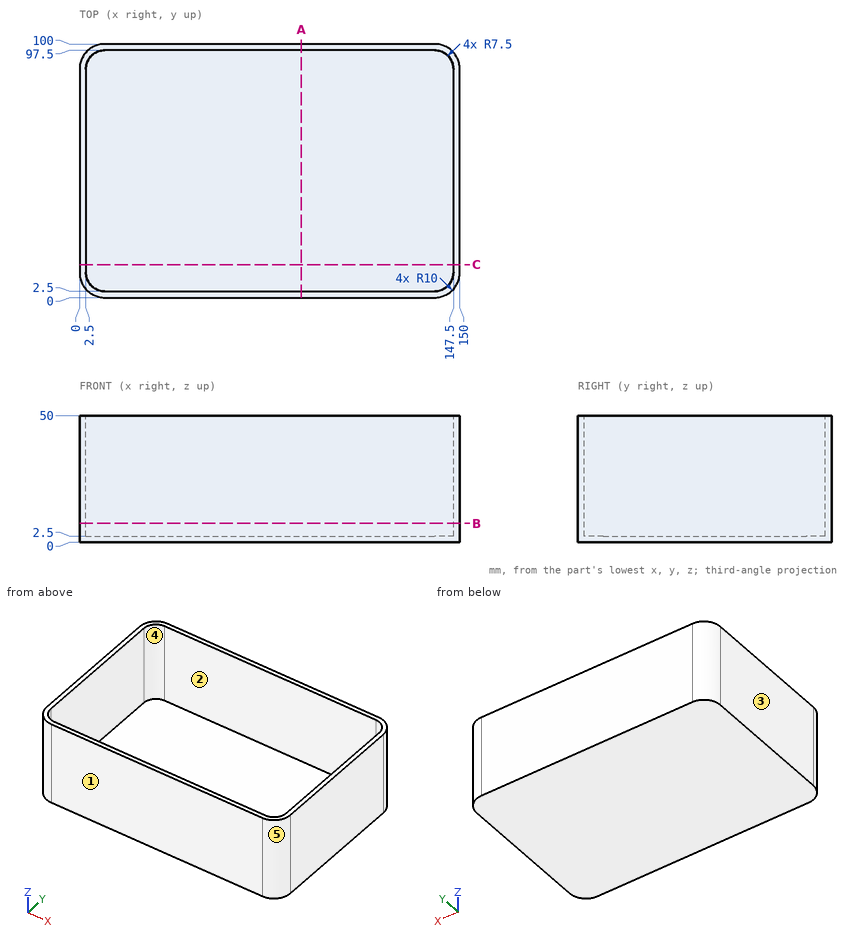
Here's the drawing with two shaded views (mm, measured from the low corner). I have some questions. A direction names the side the tool comes from. Round coordinates to 2 decimals unless told otherwise and drop trailing zeros. Order: outer loops, then holes, each group sorted by start corner. A loop starts at its lowest first (then second) coordinate and runs counter-clockwise, first axis right, second up. Notation, with made-up numbers: M 70,65 L 107,65 A18 cw 107,82 Z; hole C 23,67 d6. An arc over 180 degrees is marked long. Answer in a Markdown table with one row per item.
Item 1: For the marked faces 4 and 5, which set-ups out of +Z, -Z, +X, -X, +Y, -Y let a thin tool reach every point of the face, with its end or its side?
A:
| item | result |
|---|---|
| face 4 | +Z |
| face 5 | +Z, -Z, +X, -Y |
Item 2: Imagine slicing it at B-B, the plane z = 7.5. Write out the boundary of the cut face in (x, y), and give its area (3 significant figures).
A:
| item | result |
|---|---|
| outline | M 0,10 A10 ccw 10,0 L 140,0 A10 ccw 150,10 L 150,90 A10 ccw 140,100 L 10,100 A10 ccw 0,90 Z; hole M 2.5,10 A7.5 ccw 10,2.5 L 140,2.5 A7.5 ccw 147.5,10 L 147.5,90 A7.5 ccw 140,97.5 L 10,97.5 A7.5 ccw 2.5,90 Z |
| area | 1,190 mm2 |
Item 3: If I drill on L1, parallel to Y at x = 39, z = 26; L2, parallel to X at y = 79.5, z = 30; L3, parallel to Z at x = 118, y = 58, over which ranges is the centre line in solid material (lowest first)? Write a range as from..to.
A:
| item | result |
|---|---|
| L1 | y = 0..2.5, 97.5..100 |
| L2 | x = 0..2.5, 147.5..150 |
| L3 | z = 0..2.5 |
Item 4: Thinking about a two-plate mould opening in X: for the marked faces 1, 2 and 3, which applies, +X half, -X half, draft (parallel to the pull), parting line (faces both ways), or undercut?
A:
| item | result |
|---|---|
| face 1 | draft |
| face 2 | undercut |
| face 3 | -X half |
Item 5: I'm going to push flat-ended pins straight in: pin 1 (8 mm diameter, centred on x = 24, y = 17.5, fed in from +Z); pin 2 (10 mm diameter, centred on x = 77, y = 80.5, fed in from -Z). Where does each tip first touch, or does it pass through?
A:
| item | result |
|---|---|
| pin 1 | stops at z = 2.5 |
| pin 2 | stops at z = 0 |
Item 6: Imagine slicing it at A-A, the plane x = 87.5. Write out the boundary of the cut face in (y, z), and give its area (4 significant figures).
A:
| item | result |
|---|---|
| outline | M 0,0 L 100,0 L 100,50 L 97.5,50 L 97.5,2.5 L 2.5,2.5 L 2.5,50 L 0,50 Z |
| area | 487.5 mm2 |
Item 7: Imagine slicing it at C-C, the plane y = 13. Write out the boundary of the cut face in (x, z), and give its area (4 significant figures).
A:
| item | result |
|---|---|
| outline | M 0,0 L 150,0 L 150,50 L 147.5,50 L 147.5,2.5 L 2.5,2.5 L 2.5,50 L 0,50 Z |
| area | 612.5 mm2 |
